Solid Edge part; units mm, degrees
sketch "Sketch1" plane through (0, 0, 0) normal (0, -1, 0) x (1, 0, 0)
  circle A0 centre (0, 0) radius 9.5
  circle A1 centre (0, 0) radius 3
extrude "Protrusion1" add sketch "Sketch1" along normal blind 6
sketch "Sketch2" plane through (0, 0, 0) normal (0, 1, 0) x (-1, 0, 0)
  circle A0 centre (0, 0) radius 8.25
  circle A1 centre (0, 0) radius 4.75
extrude "ExtrudedCutout_1" cut sketch "Sketch2" against normal blind 0.5
sketch "Sketch3" plane through (0, -6, 0) normal (0, -1, 0) x (1, 0, 0)
  circle A0 centre (0, 0) radius 8.25
  circle A1 centre (0, 0) radius 4.75
extrude "ExtrudedCutout_4" cut sketch "Sketch3" against normal blind 0.5
properties material "Steel"
Here's how the part is built. I have some questions about the finished solid (model axes, mm). A direction names the side the tool comes from. Coordinates: 2 decimals unless noted, no trailing zeros. Order: outer loops, then holes, each group sorted by start corner. A loop starts at its lowest first (then second) coordinate and runs counter-clockwise, first axis right, second up. Notation, with made-up numbers: M -15.5,52.5 L 21.5,52.5 A19 ccw 21.5,67.5 Z; hole C 39.25,83 d5. An arc over 180 degrees is marked long. Answer as a JSON object with one key per item and string values. Group by question number.
(1) Suppose I cut it at C-C, the plane y = -1.8. Please give me the cut outline in (x, z), then the cut area to 3 significant figures.
(2) If we mould it in two halves opening along X, with no side actions, what happens to faces 4 (the face through (-3, -3, 0)), 5 (the face through (8, -6, 3)), 6 (the face through (-4, -0.5, 4)), 7 (the face through (4.38, -2.96, 8.43))? For each: released by +X, released by -X, zero draft, split by the parting line, or undercut.
(3) For pin 1 (3 mm diameter, centred on y = -5, z = -7.5, fed in from +X); pin 2 (3 mm diameter, centred on y = -2.5, z = -2.5, fed in from -X), each with a flat end and sliding along its axis, tell me the tip position at first contact or that it passes through.
(4) Which directions (+Z, -Z, +X, -X, +Y, -Y) give clear straight access to the entire face, cutting with the end or side of a thin tool? Please do faces 1 (the face through (-4, -5.5, -4)), 2 (the face through (-2.192, -0.246, -4.214)), 3 (the face through (-1, -6, -3)).
(5) Suppose I cut it at B-B, the plane z = 0. Please give me the cut outline in (x, y), then the cut area to 3 significant figures.
(6) I need wall thicknesses on probe 1 along Z at (x, y) = (0, -0.3); probe 2 along Z at (x, y) = (-3.5, -5.6); probe 3 along Z at (x, y) = (1.25, -0.4). Which ranges of each line are inside material? Lowest first, please.
(7) Suppose I cut it at D-D, the plane x = -3.5. Please give me the cut outline in (y, z), then the cut area to 3 significant figures.
(8) Suppose I cut it at A-A, the plane x = 0. Please give me the cut outline in (y, z), then the cut area to 3 significant figures.
Values found:
{
 "1": {"outline": "C 0,0 d19; hole C 0,0 d6", "area": "255 mm^2"},
 "2": {"face 4": "undercut", "face 5": "zero draft", "face 6": "undercut", "face 7": "split by the parting line"},
 "3": {"pin 1": "stops at x = 7.37", "pin 2": "stops at x = -9.45"},
 "4": {"face 1": "-Y", "face 2": "+Y", "face 3": "+Z, -Z, +X, -X, -Y"},
 "5": {"outline": "M -9.5,-6 L -8.25,-6 L -8.25,-5.5 L -4.75,-5.5 L -4.75,-6 L -3,-6 L -3,0 L -4.75,0 L -4.75,-0.5 L -8.25,-0.5 L -8.25,0 L -9.5,0 Z; M 3,-6 L 4.75,-6 L 4.75,-5.5 L 8.25,-5.5 L 8.25,-6 L 9.5,-6 L 9.5,0 L 8.25,0 L 8.25,-0.5 L 4.75,-0.5 L 4.75,0 L 3,0 Z", "area": "71.0 mm^2"},
 "6": {"probe 1": "z = -9.5 to -8.25, -4.75 to -3, 3 to 4.75, 8.25 to 9.5", "probe 2": "z = -8.83 to -7.47, -3.21 to 3.21, 7.47 to 8.83", "probe 3": "z = -9.42 to -8.15, -4.58 to -2.73, 2.73 to 4.58, 8.15 to 9.42"},
 "7": {"outline": "M -6,-8.83 L 0,-8.83 L 0,-7.47 L -0.5,-7.47 L -0.5,-3.21 L 0,-3.21 L 0,3.21 L -0.5,3.21 L -0.5,7.47 L 0,7.47 L 0,8.83 L -6,8.83 L -6,7.47 L -5.5,7.47 L -5.5,3.21 L -6,3.21 L -6,-3.21 L -5.5,-3.21 L -5.5,-7.47 L -6,-7.47 Z", "area": "97.5 mm^2"},
 "8": {"outline": "M -6,-9.5 L 0,-9.5 L 0,-8.25 L -0.5,-8.25 L -0.5,-4.75 L 0,-4.75 L 0,-3 L -6,-3 L -6,-4.75 L -5.5,-4.75 L -5.5,-8.25 L -6,-8.25 Z; M -6,3 L 0,3 L 0,4.75 L -0.5,4.75 L -0.5,8.25 L 0,8.25 L 0,9.5 L -6,9.5 L -6,8.25 L -5.5,8.25 L -5.5,4.75 L -6,4.75 Z", "area": "71.0 mm^2"}
}
